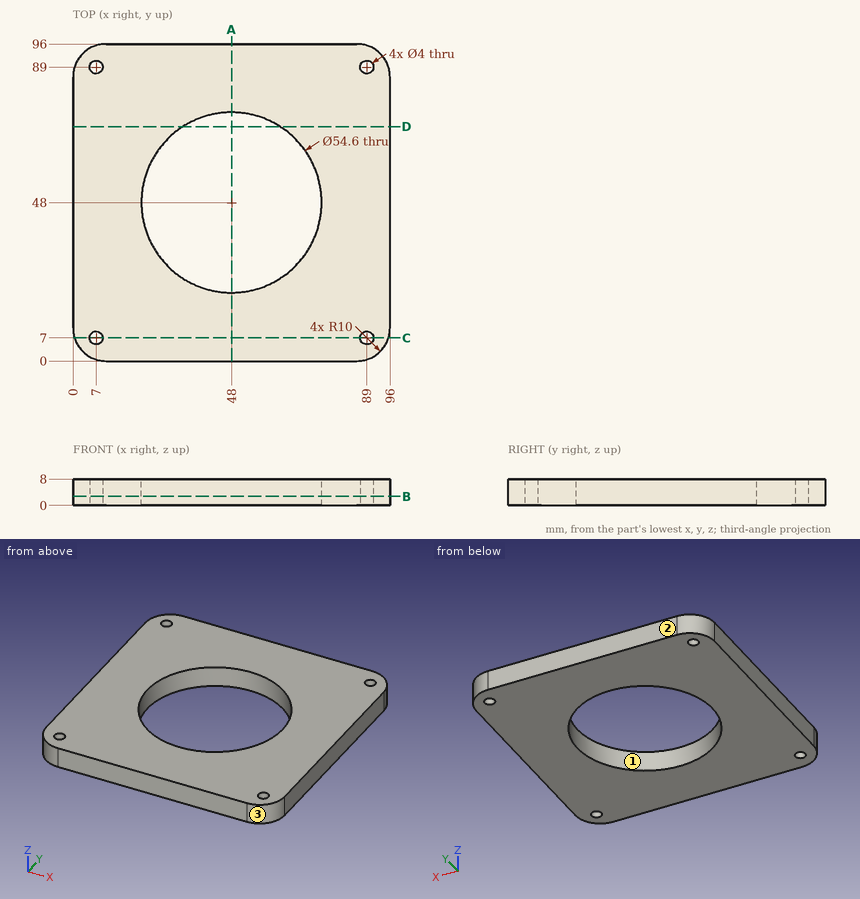
Input: dimensioned drawing with shaded views. Units: mm. Origin: part minimum x, y, z. Coordinates: 2 decimals unless noted, no trailing zeros. Order: outer loops, then holes, each group sorted by start corner. A loop starts at its lowest first (then second) coordinate and runs counter-clockwise, first axis right, second up. Notation, with made-up numbers: (28.25, 48) - (71.25, 48) arc R10 cw to (71.25, 54) - close; hole circle Ø1 at (55.25, 57). An arc over 180 degrees is marked (long way). Put each result on its own line as item: value.
1. Cut plane C-C on y = 7. Return the cut outline in (x, z), then the cut area to 3 significant figures.
Report:
outline: (0.46, 0) - (5, 0) - (5, 8) - (0.46, 8) - close; (9, 0) - (87, 0) - (87, 8) - (9, 8) - close; (91, 0) - (95.54, 0) - (95.54, 8) - (91, 8) - close
area: 697 mm2
2. Cut plane B-B on z = 2.75. Return the cut outline in (x, y).
Report:
outline: (0, 10) arc R10 ccw to (10, 0) - (86, 0) arc R10 ccw to (96, 10) - (96, 86) arc R10 ccw to (86, 96) - (10, 96) arc R10 ccw to (0, 86) - close; hole circle Ø4 at (7, 7); hole circle Ø4 at (7, 89); hole circle Ø54.6 at (48, 48); hole circle Ø4 at (89, 7); hole circle Ø4 at (89, 89)
3. Line query: line 1 along Y through (x, z) = (48, 4.25); line 2 along Y through (x, z) = (89, 1.5); line 3 along Y through (x, z) = (68.5, 1). Output: solid intervals per line, ascending.
Report:
line 1: y = 0 to 20.7, 75.3 to 96
line 2: y = 0.46 to 5, 9 to 87, 91 to 95.54
line 3: y = 0 to 29.97, 66.03 to 96
4. Draft query along X for the marked faces 1, 2 and 3. Return one class per face: pulls with the +X half, pulls with the -X half, needs draft (parallel to the pull), parting line crosses it, or undercut.
Report:
face 1: undercut
face 2: needs draft
face 3: pulls with the +X half
5. Cut plane A-A on x = 48. Return the cut outline in (y, z).
Report:
outline: (0, 0) - (20.7, 0) - (20.7, 8) - (0, 8) - close; (75.3, 0) - (96, 0) - (96, 8) - (75.3, 8) - close
6. Cut plane D-D on y = 71. Return the cut outline in (x, z), then the cut area to 3 significant figures.
Report:
outline: (0, 0) - (33.29, 0) - (33.29, 8) - (0, 8) - close; (62.71, 0) - (96, 0) - (96, 8) - (62.71, 8) - close
area: 533 mm2
